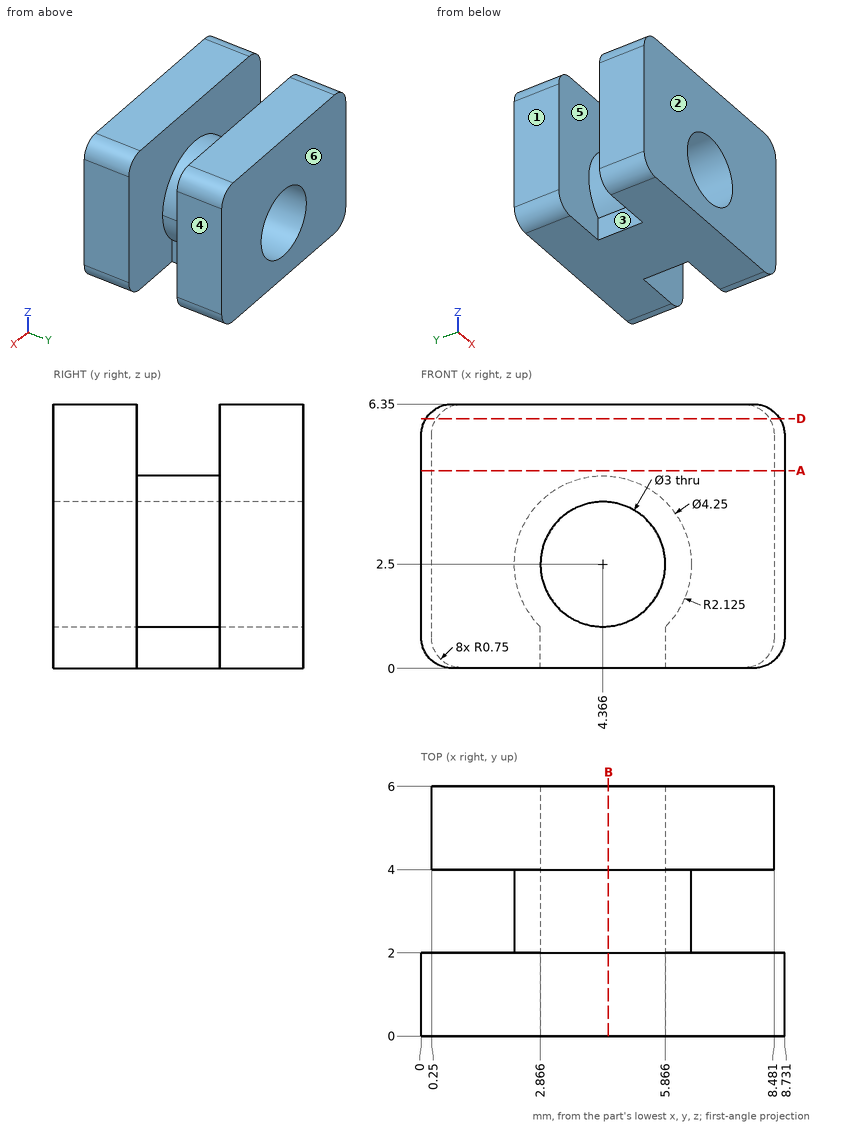
Print and shaded views of the part. All mm, measured from the part's lowest x, y and z. A direction names the side the tool comes from. Coordinates: 2 decimals unless noted, no trailing zeros. Order: outer loops, then holes, each group sorted by start corner. A loop starts at its lowest first (then second) coordinate and runs counter-clockwise, first axis right, second up. Notation, with made-up numbers: M -8,43.5 L 23,43.5 A7 ccw 23,49.5 Z; hole C 73,-13 d6. An arc over 180 degrees is marked long. One line per question, with ' | ' between items. Start each with the question number.
Q1. Saw through at A-A (z = 4.75). List the corners of the cut face in (x, y).
Q2. Probe L1, parallel to Y at x = 1.5, z = 5; L2, parallel to X at y = 5.5, z = 4.75; L3, parallel to X at y = 1, z = 2.75 (1 decimal). List the from-to ranges inside material, lowest first. Write a range as from..to.
Q3. Saw through at B-B (x = 4.5). List the corners of the cut face in (y, z).
Q4. Two-plate mould, pull along Y, no slides. Class the marked faces 3, 4, 5 and 6: +Y half, -Y half, draft (parallel to the pull), parting line (faces both ways), or undercut.
Q5. 3-axis set-ups, long thin cutter, end or side, ignore diameter. For the marked faces 1 and 2: which of +Z, -Z, +X, -X, +Y, -Y reach the whole face in a straight line?
Q6. Flat gauge pins, fed straight in: pin 1 Ø2 at (y, z) = (5, 2.5) entering from +X; pin 2 Ø2.5 at (x, z) = (4.37, 2.5) entering from -Y; pin 3 Ø2 at (y, z) = (4.5, 1) entering from -X; pin 4 Ø0.5 at (y, z) = (3, 0.5) entering from +X. Where does each tip first touch, or does it go through?
Q7. Saw through at D-D (z = 6). List the corners of the cut face in (x, y) (1 decimal).
Check values:
1) outline: M 0,0 L 8.73,0 L 8.73,2 L 0,2 Z; M 0.25,4 L 8.48,4 L 8.48,6 L 0.25,6 Z
2) L1: y = 0..2, 4..6 | L2: x = 0.25..8.48 | L3: x = 0..2.9, 5.8..8.7
3) outline: M 0,0 L 6,0 L 6,1.01 L 0,1.01 Z; M 0,3.99 L 6,3.99 L 6,6.35 L 4,6.35 L 4,4.62 L 2,4.62 L 2,6.35 L 0,6.35 Z
4) face 3: undercut | face 4: draft | face 5: undercut | face 6: +Y half
5) face 1: +Z, -Z, -X, +Y | face 2: +Z, -Z, +X, -X, -Y
6) pin 1: stops at x = 8.48 | pin 2: passes through | pin 3: stops at x = 0.25 | pin 4: stops at x = 5.87
7) outline: M 0.1,0 L 8.6,0 L 8.6,2 L 0.1,2 Z; M 0.4,4 L 8.4,4 L 8.4,6 L 0.4,6 Z
